Read the model definition and answer for the solid it produces. Units are mm, in the model's axes. A direction names the side the tool comes from. Coordinates: 2 decimals unless noted, no trailing zeros. Loops run counter-clockwise (first coordinate to the right, second up) from the corner with the lowest first, then second, coordinate; pieces in that order, holes last. Notation, with made-up numbers: M 45,51 L 54,51 A24 ccw 54,61 Z; hole C 24.25,2 d2. An arc over 180 degrees is marked long. Put each result on its own line as item: value.
from build123d import *

# Parameters (mm, degrees)
WALL_DEPTH                = 16
ROOF_START                = 16
ROOF_DEPTH                = 3.175
F_2_56_TAPPED_HOLE1_D     = 1.778
F_2_56_TAPPED_HOLE1_DEPTH = 5.73
F_2_56_TAPPED_HOLE1_TIP   = 0.53416509
BOSS_EXTRUDE1_DEPTH       = 1.5875
CUT_EXTRUDE3_DEPTH        = 2
FILLET1_R                 = 1.5875
RAIL_CUT_DEPTH            = 56.855288749
RAIL_CUT_DEPTH_BACK       = 28
SKETCH4_W                 = 2
SKETCH4_H                 = 3.175
FILLET2_R                 = 1


with BuildPart() as part:
    # MainSketch → Wall (new body)
    with BuildSketch(Plane(origin=(0, 0, 0), x_dir=(1, 0, 0), z_dir=(0, 1, 0))):
        Polygon((-31, -2.5), (0, -2.5), (0, 0), (-33.5, 0), (-33.5, -39), (0, -39), (0, -36.5), (-31, -36.5), align=None)
    extrude(amount=WALL_DEPTH)

    # MainSketch<3> → Roof (add)
    with BuildSketch(Plane(origin=(0, 0, 0), x_dir=(1, 0, 0), z_dir=(0, 1, 0)).offset(ROOF_START)):
        Polygon((0, -12), (0, 0), (-33.5, 0), (-33.5, -39), (0, -39), (0, -27), (-5.5, -27), (-5.5, -12), align=None)
    extrude(amount=ROOF_DEPTH)

    # #2-56 Tapped Hole1
    with Locations(Plane(origin=(-16.75, 0, 37.75), x_dir=(0, 0, -1), z_dir=(0, -1, 0))):
        with Locations((0, 0), (36.5, 0)):
            Hole(F_2_56_TAPPED_HOLE1_D / 2, depth=F_2_56_TAPPED_HOLE1_DEPTH)
            with Locations((0, 0, -(F_2_56_TAPPED_HOLE1_DEPTH + F_2_56_TAPPED_HOLE1_TIP / 2))):  # 118° drill point
                Cone(0, F_2_56_TAPPED_HOLE1_D / 2, F_2_56_TAPPED_HOLE1_TIP, mode=Mode.SUBTRACT)

    # Sketch3 → Boss-Extrude1 (add)
    with BuildSketch(Plane(origin=(0, 0, 0), x_dir=(0, 0, -1), z_dir=(1, 0, 0))):
        Polygon((-28, 17), (-28, 16), (-36.5, 16), (-36.5, 0), (-37.5, 0), (-37.5, 17), align=None)
    extrude(amount=BOSS_EXTRUDE1_DEPTH)

    # Sketch3<3> → Cut-Extrude3 (cut)
    with BuildSketch(Plane(origin=(0, 0, 0), x_dir=(0, 0, -1), z_dir=(1, 0, 0))):
        Polygon((-11.5, 16), (-11.5, 17.5), (-1, 17.5), (-1, 0), (-2.5, 0), (-2.5, 16), align=None)
    extrude(amount=-CUT_EXTRUDE3_DEPTH, mode=Mode.SUBTRACT)

    # Fillet1
    fillet1_edges = [part.edges().sort_by_distance(p)[0] for p in [
        (0.79375, 17, 37.5),
        (1.5875, 16.5, 28),
        (-1, 17.5, 1),
        (-2, 16.75, 11.5),
    ]]
    fillet(fillet1_edges, radius=FILLET1_R - 0.0001)  # a hair under: the kernel refuses the full size

    # Sketch4 → rail cut (cut, two sides: drawn at the far end of the back side and taken through both)
    with BuildSketch(Plane.ZY.offset(33.5).offset(-RAIL_CUT_DEPTH_BACK)):
        with Locations((1, 14.5875)):
            Rectangle(SKETCH4_W, SKETCH4_H)
        with Locations((38, 14.5875)):
            Rectangle(SKETCH4_W, SKETCH4_H)
    extrude(amount=RAIL_CUT_DEPTH + RAIL_CUT_DEPTH_BACK, mode=Mode.SUBTRACT)

    # Fillet2
    fillet2_edges = [part.edges().sort_by_distance(p)[0] for p in [
        (-5.5, 16.175, 1),
        (-5.5, 13, 1),
        (-5.5, 13, 38),
        (-5.5, 16.175, 38),
        (-31, 8, 2.5),
        (-31, 8, 36.5),
    ]]
    fillet(fillet2_edges, radius=FILLET2_R)


solid = part.part
1) Which of the six approach directions +Z, -Z, +X, -X, +Y, -Y give full straight-line access (tool end or side, diameter ignored) to faces 5 (the flat face through (-5.5, 18, 20)), 6 (the cylindrical face through (0.8, 16.55, 37.02)), 7 (the flat face through (-20, 16.175, 38)), 8 (the flat face through (-31, 8, 20))?
Answer list:
face 5: +X, +Y, -Y
face 6: +Z, +X, +Y
face 7: +Z, -X
face 8: +X, -Y
2) Straight lines are drawn through the part: line 1 (Z direction, x = -16.75, y = 2.4); line 2 (Z direction, x = -14, y = 7); line 3 (Z direction, x = -1.5, y = 12). For each, find the intervals that lie inside material, in ascending order. Write a range as [from, to].
Answer list:
line 1: z = [0, 0.36], [2.14, 2.5], [36.5, 36.86], [38.64, 39]
line 2: z = [0, 2.5], [36.5, 39]
line 3: z = [0, 1], [36.5, 39]
3) Determine the mould class of faces 1 (the flat face through (-17, 19.175, 19)), 2 (the flat face through (1, 8, 37.5)), 3 (the cylindrical face through (-1.52, 16.76, 11.05)), 4 (the cylindrical face through (1.11, 16.49, 28.45)) for opening direction Z: released by +Z, released by -Z, zero draft, split by the parting line, or undercut.
Answer list:
face 1: zero draft
face 2: released by +Z
face 3: undercut
face 4: released by -Z
4) Find section A-A, the plane y = 1.5. Write down the section's boundary in (x, z).
Answer list:
outline: M -33.5,0 L 0,0 L 0,1 L -2,1 L -2,2.5 L -30,2.5 A1 cw -31,3.5 L -31,35.5 A1 cw -30,36.5 L 1.59,36.5 L 1.59,37.5 L 0,37.5 L 0,39 L -33.5,39 Z; hole C -16.75,1.25 d1.78; hole C -16.75,37.75 d1.78
5) Given pin 1 Ø0.6 at (y, z) = (14.5, 0.5) entering from -X; pin 2 Ø5 at (x, y) = (-6, 2) entering from -Z; pin 3 Ø2.5 at (x, y) = (-16.5, 14.5) entering from +Z; pin 4 Ø3.5 at (y, z) = (17, 16) entering from +X, each flat-ended and moving along its own axis, determine where each tip first touches the part or whether it passes through.
Answer list:
pin 1: stops at x = -5.5
pin 2: stops at z = 0
pin 3: stops at z = 37
pin 4: stops at x = -5.5
6) Find section C-C, the plane x = -20. Write down the section's boundary in (y, z) (3 decimals), plus the area to 3 significant figures.
Answer list:
outline: M 0,0 L 13,0 L 13,2 L 16.175,2 L 16.175,0 L 19.175,0 L 19.175,39 L 16.175,39 L 16.175,37 L 13,37 L 13,39 L 0,39 L 0,36.5 L 16,36.5 L 16,2.5 L 0,2.5 Z
area: 191 mm^2
7) Find section B-B, the plane z = 34. Write down the section's boundary in (x, y) (1 decimal).
Answer list:
outline: M -33.5,0 L -31,0 L -31,16 L 1.6,16 L 1.6,17 L 0,17 L 0,19.2 L -33.5,19.2 Z
8) Find section D-D, the plane y = 7.25. Write down the section's boundary in (x, z).
Answer list:
outline: M -33.5,0 L 0,0 L 0,1 L -2,1 L -2,2.5 L -30,2.5 A1 cw -31,3.5 L -31,35.5 A1 cw -30,36.5 L 1.59,36.5 L 1.59,37.5 L 0,37.5 L 0,39 L -33.5,39 Z
